from build123d import *

# Parameters (mm, degrees)
SKETCH2_R           = 18.5
SKETCH2_R_2         = 13.5
BOSS_EXTRUDE2_DEPTH = 5
BOSS_EXTRUDE3_DEPTH = 5
SKETCH4_R           = 11
BOSS_EXTRUDE4_DEPTH = 5
SKETCH5_R           = 8
CUT_EXTRUDE1_DEPTH  = 5
BOSS_EXTRUDE5_DEPTH = 5
BOSS_EXTRUDE6_DEPTH = 5


with BuildPart() as part:
    # Sketch2 → Boss-Extrude2 (new body)
    with BuildSketch(Plane(origin=(0, 0, 0), x_dir=(1, 0, 0), z_dir=(0, 1, 0))):
        with Locations(Location((0, 0, 0), (0, 0, 270))):
            Circle(SKETCH2_R)
        with Locations(Location((0, 0, 0), (0, 0, 270))):
            Circle(SKETCH2_R_2, mode=Mode.SUBTRACT)
    extrude(amount=BOSS_EXTRUDE2_DEPTH)

    # Sketch3 → Boss-Extrude3 (add)
    with BuildSketch(Plane(origin=(0, 5, 0), x_dir=(1, 0, 0), z_dir=(0, 1, 0))):
        Polygon((25.460427034, 3.126984488), (25.460427034, -2.892028048), (18.27255247, -2.892028048), (18.27255247, 2.892028048), align=None)
    extrude(amount=-BOSS_EXTRUDE3_DEPTH)

    # Sketch4 → Boss-Extrude4 (add)
    with BuildSketch(Plane(origin=(0, 5, 0), x_dir=(1, 0, 0), z_dir=(0, 1, 0))):
        with Locations((36, 0.11747822)):
            Circle(SKETCH4_R)
    extrude(amount=-BOSS_EXTRUDE4_DEPTH)

    # Sketch5 → Cut-Extrude1 (cut)
    with BuildSketch(Plane(origin=(0, 5, 0), x_dir=(1, 0, 0), z_dir=(0, 1, 0))):
        with Locations(Location((36, 0.11747822, 0), (0, 0, 270))):
            Circle(SKETCH5_R)
    extrude(amount=-CUT_EXTRUDE1_DEPTH, mode=Mode.SUBTRACT)

    # Sketch6 → Boss-Extrude5 (add)
    with BuildSketch(Plane(origin=(0, 5, 0), x_dir=(1, 0, 0), z_dir=(0, 1, 0))):
        Polygon((38.256533955, 10.883538526), (3.795079834, 18.106555969), (18.27255247, 2.892028048), (25.419311952, 3.125640523), align=None)
    extrude(amount=-BOSS_EXTRUDE5_DEPTH)

    # Sketch7 → Boss-Extrude6 (add)
    with BuildSketch(Plane(origin=(0, 5, 0), x_dir=(1, 0, 0), z_dir=(0, 1, 0))):
        Polygon((38.32675057, -10.633625527), (3.913171414, -18.081401757), (18.27255247, -2.892028048), (25.419694143, -2.892028048), align=None)
    extrude(amount=-BOSS_EXTRUDE6_DEPTH)


solid = part.part
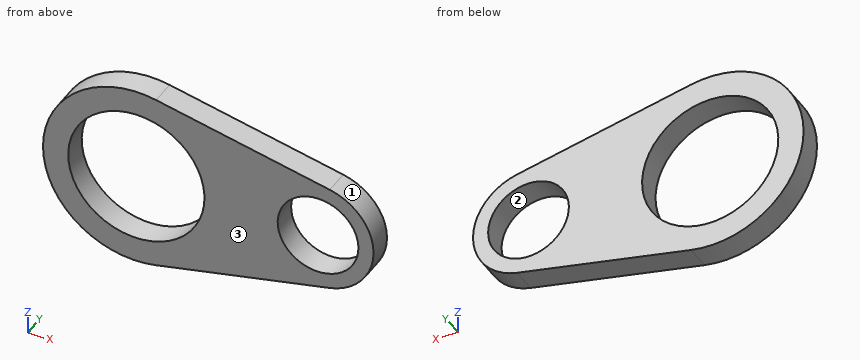
Read the model definition and answer for the solid it produces. Units are mm, in the model's axes. Face numbers are marked on the shaded views. Give positions to 0.01 mm unless a question says otherwise; leave off trailing zeros. Write each loop counter-clockwise with the first axis right and the second up, starting at its lowest first coordinate (ties: lowest second). Pieces come first, ordered by that corner, then holes. Notation, with made-up numbers: (-27.75, 81) -> (30.25, 81) arc R24 ccw to (30.25, 114) -> close; hole circle Ø9 at (71, -24). An arc over 180 degrees is marked (long way). Answer as a JSON object with one key per item and string values. Group by question number.
1) Each of these flat-tipped pins is pushed along its axis until it touches: P1, Ø6, axis at x = 7.5, z = 4.5, coming from the +Y side; P2, Ø1, axis at y = 3.5, z = -6.5, coming from the +X side; P3, Ø2, axis at x = 28, y = 3.5, coming from the -Z side. Where does it stop, or does it pass through?
2) Find section A-A (x = 0). Write down the section's boundary in (y, z), and give its area (3 significant figures).
3) Consider L1, parallel to X at y = 2.1, z = 0; L2, parallel to X at y = 1.15, z = -6.5; L3, parallel to Z at x = 41, y = 2.95. Determine where each line is inside the solid, lowest interval first. Write a range as from..to.
4) The mould has two halves that part along X. Classify the marked faces 1, 2 and 3: +X half, -X half, draft (parallel to the pull), parting line (faces both ways), or undercut.
5) Find section B-B (z = 0). Write down the section's boundary in (x, y), and give its area (3 significant figures).
6) Find section C-C (y = 3.2). Write down the section's boundary in (x, z), and give its area (3 significant figures).
7) Find section D-D (z = -11.5). Write down the section's boundary in (x, y).
Values follow:
{
 "1": {"P1": "passes through", "P2": "stops at x = 45.29", "P3": "stops at z = -13.24"},
 "2": {"outline": "(0, -18.5) -> (5, -18.5) -> (5, -13.5) -> (0, -13.5) -> close; (0, 13.5) -> (5, 13.5) -> (5, 18.5) -> (0, 18.5) -> close", "area": "50.0 mm2"},
 "3": {"L1": "x = -18.5..-13.5, 13.5..28, 44..47", "L2": "x = -17.32..-11.83, 11.83..31.18, 40.82..44.96", "L3": "z = -9.92..-6.36, 6.13..9.68"},
 "4": {"face 1": "+X half", "face 2": "undercut", "face 3": "draft"},
 "5": {"outline": "(-18.5, 0) -> (-13.5, 0) -> (-13.5, 5) -> (-18.5, 5) -> close; (13.5, 0) -> (28, 0) -> (28, 5) -> (13.5, 5) -> close; (44, 0) -> (47, 0) -> (47, 5) -> (44, 5) -> close", "area": "113 mm2"},
 "6": {"outline": "(3.8, -18.11) -> (38.26, -10.88) arc R11 ccw to (38.33, 10.63) -> (3.91, 18.08) arc R18.5 ccw (long way) to start; hole circle Ø27 at (0, 0); hole circle Ø16 at (36, -0.12)", "area": "1,040 mm2"},
 "7": {"outline": "(-14.49, 0) -> (-7.07, 0) -> (-7.07, 5) -> (-14.49, 5) -> close; (7.07, 0) -> (35.32, 0) -> (35.32, 5) -> (7.07, 5) -> close"}
}
